```python
from build123d import *

# Parameters (mm, degrees)
SKETCH1_W           = 100
SKETCH1_H           = 150
BOSS_EXTRUDE1_DEPTH = 100
CUT_EXTRUDE1_DEPTH  = 50
CUT_EXTRUDE2_DEPTH  = 207.155281281


with BuildPart() as part:
    # Sketch1 → Boss-Extrude1 (new body)
    with BuildSketch(Plane.XY):
        with Locations((50, 75)):
            Rectangle(SKETCH1_W, SKETCH1_H)
    extrude(amount=-BOSS_EXTRUDE1_DEPTH)

    # Sketch2 → Cut-Extrude1 (cut)
    with BuildSketch(Plane.XZ):
        Polygon((25, 0), (50, -45), (75, 0), align=None)
    extrude(amount=-CUT_EXTRUDE1_DEPTH, mode=Mode.SUBTRACT)

    # Sketch3 → Cut-Extrude2 (cut, through all)
    with BuildSketch(Plane.ZY):
        Polygon((0, 125), (-20, 125), (-20, 105), (-40, 105), (-40, 85), (-20, 85), (-20, 65), (0, 65), align=None)
    extrude(amount=-CUT_EXTRUDE2_DEPTH, mode=Mode.SUBTRACT)


solid = part.part
```
For this review, take the finished solid that the model builds, in its own axes (mm). A direction names the side the tool comes from. Give positions to 0.01 mm unless a question says otherwise; leave off trailing zeros. Write each loop counter-clockwise with the first axis right and the second up, starting at its lowest first coordinate (ties: lowest second). Pieces come first, ordered by that corner, then holes. Notation, with made-up numbers: M 28.25,9 L 41.25,9 A22 ccw 41.25,43 Z; hole C 13.5,47 d3. An arc over 180 degrees is marked long. Answer as a JSON object with one key per item and string values. Group by question number.
Item 1: For probe 1 along Y at (x, z) = (42, -9); probe 2 along Y at (x, z) = (19.5, -17.5); probe 3 along Z at (x, y) = (35, 68.5), list the stretches that pass through material, from the lowest coordinate up. Write a range as [from, to].
Item 2: Consider section C-C on y = 20.5. Write out the cut boundary in (x, z), plus the area to 4 significant figures.
Item 3: Draft analysis for pull direction Y (two halves, no side actions). For faces 4 (the flat face through (49, 65, -10)), 5 (the flat face through (49, 0, -49)), 6 (the flat face through (0, 74, -49)), 7 (the flat face through (49, 150, -49)), state which applies: +Y half, -Y half, draft (parallel to the pull), parting line (faces both ways), or undercut.
Item 4: Tool access review of faces 1 (the flat face through (49, 105, -30)), 2 (the flat face through (62.325, 24.65, -22.815)), 3 (the flat face through (49, 76, -100)): name each direction out of +Z, -Z, +X, -X, +Y, -Y from which nothing blocks a thin tool from reaching the whole face with its end or side.
Item 5: Consider section B-B on x = 63. Write out the cut boundary in (y, z).
Item 6: Consider section A-A on z = -34. Write out the cut boundary in (x, y).
Item 7: For pin 1 Ø6 at (x, y) = (39.5, 99.5) entering from +Z, flat-tipped, find the tip position at first contact; note if it passes through.
Item 8: Consider section D-D on z = -23.5. Write out the cut boundary in (x, y), plus the area to 3 significant figures.
Check result:
{
 "1": {"probe 1": "y = [50, 65], [125, 150]", "probe 2": "y = [0, 65], [125, 150]", "probe 3": "z = [-100, -20]"},
 "2": {"outline": "M 0,-100 L 100,-100 L 100,0 L 75,0 L 50,-45 L 25,0 L 0,0 Z", "area": "8,875 mm^2"},
 "3": {"face 4": "undercut", "face 5": "-Y half", "face 6": "draft", "face 7": "+Y half"},
 "4": {"face 1": "+Z, +X, -X", "face 2": "+Z, -Y", "face 3": "-Z, +X, -X, +Y, -Y"},
 "5": {"outline": "M 0,-100 L 150,-100 L 150,0 L 125,0 L 125,-20 L 105,-20 L 105,-40 L 85,-40 L 85,-20 L 65,-20 L 65,0 L 50,0 L 50,-21.6 L 0,-21.6 Z"},
 "6": {"outline": "M 0,0 L 43.89,0 L 43.89,50 L 56.11,50 L 56.11,0 L 100,0 L 100,85 L 0,85 Z; M 0,105 L 100,105 L 100,150 L 0,150 Z"},
 "7": {"pin 1": "stops at z = -40"},
 "8": {"outline": "M 0,0 L 38.06,0 L 38.06,50 L 61.94,50 L 61.94,0 L 100,0 L 100,85 L 0,85 Z; M 0,105 L 100,105 L 100,150 L 0,150 Z", "area": "11,800 mm^2"}
}
